CAD build for the part. Positions are in the model's coordinates, mm. Give positions to 0.01 mm unless a question says otherwise; leave off trailing zeros. Write each loop counter-clockwise with the first axis right and the second up, starting at its lowest first coordinate (ties: lowest second). Pieces come first, ordered by that corner, then holes. Notation, with made-up numbers: M 59.25,-4 L 77.25,-4 A27 cw 77.25,22 Z; hole C 2,6 d8. An arc over 180 degrees is marked long. One line per question, with ' | ' between items. Start each with the question number.
1. Wall check: L1, parallel to Y at x = -65, z = 2.1; L2, parallel to Y at x = -68.5, z = 1; L3, parallel to X at y = 59.5, z = 1. Give the ranges that are in metal, low to high.
2. Cut at C-C, the plane x = -58.5. Write the cut outline in (y, z).
3. Cut at B-B, the plane z = 5. Count the separate pieces of the cut face and the enclosed holes in it, then the cut area to 3 significant figures.
4. Cut at D-D, the plane y = 65. Write the cut outline in (x, z).
5. Flat gauge pins, fed straight in: pin 1 (1.5 mm diameter, centred on y = 38, z = 5, fed in from +X); pin 2 (5 mm diameter, centred on x = 65, y = -65, fed in from +Z); pin 3 (3 mm diameter, centred on x = -57.5, z = 5, fed in from -Y); pin 4 (1.5 mm diameter, centred on y = 2, z = 4, fed in from -X). Where does each tip first touch, or does it go through?
6. Cut at A-A, the plane y = 0. Write the cut outline in (x, z).
```python
from build123d import *

# Parameters (mm, degrees)
F0_R     = 4.25
F0_R_2   = 2.6
F1_DEPTH = 6
F2_R     = 20


with BuildPart() as f1:
    # F0 (on Top) → F1 (new body)
    with BuildSketch(Plane.XY):
        with BuildLine():
            Line((56.161165, 73.838835), (25.393825, 43.071495))
            ThreePointArc((25.393825, 43.071495), (0, 50), (-25.393825, 43.071495))
            Line((-25.393825, 43.071495), (-56.161165, 73.838835))
            ThreePointArc((-56.161165, 73.838835), (-73.838835, 73.838835), (-73.838835, 56.161165))
            Line((-73.838835, 56.161165), (-43.071495, 25.393825))
            ThreePointArc((-43.071495, 25.393825), (-50, 0), (-43.071495, -25.393825))
            Line((-43.071495, -25.393825), (-73.838835, -56.161165))
            ThreePointArc((-73.838835, -56.161165), (-73.838835, -73.838835), (-56.161165, -73.838835))
            Line((-56.161165, -73.838835), (-25.393825, -43.071495))
            ThreePointArc((-25.393825, -43.071495), (0, -50), (25.393825, -43.071495))
            Line((25.393825, -43.071495), (56.161165, -73.838835))
            ThreePointArc((56.161165, -73.838835), (73.838835, -73.838835), (73.838835, -56.161165))
            Line((73.838835, -56.161165), (43.071495, -25.393825))
            ThreePointArc((43.071495, -25.393825), (50, 0), (43.071495, 25.393825))
            Line((43.071495, 25.393825), (73.838835, 56.161165))
            ThreePointArc((73.838835, 56.161165), (73.838835, 73.838835), (56.161165, 73.838835))
        make_face()
        with Locations((-65, -65)):
            Circle(F0_R, mode=Mode.SUBTRACT)
        with Locations((65, -65)):
            Circle(F0_R, mode=Mode.SUBTRACT)
        with Locations((-32.5, 0)):
            Circle(F0_R_2, mode=Mode.SUBTRACT)
        with Locations((-65, 65)):
            Circle(F0_R, mode=Mode.SUBTRACT)
        with Locations((32.5, 0)):
            Circle(F0_R_2, mode=Mode.SUBTRACT)
        with Locations((65, 65)):
            Circle(F0_R, mode=Mode.SUBTRACT)
    extrude(amount=F1_DEPTH)

    # F2
    f2_edges = [f1.edges().sort_by_distance(p)[0] for p in [
        (-25.393825, -43.071495, 3),
        (25.393825, -43.071495, 3),
        (43.071495, -25.393825, 3),
        (43.071495, 25.393825, 3),
        (25.393825, 43.071495, 3),
        (-25.393825, 43.071495, 3),
        (-43.071495, 25.393825, 3),
        (-43.071495, -25.393825, 3),
    ]]
    fillet(f2_edges, radius=F2_R)


solid = f1.part
```
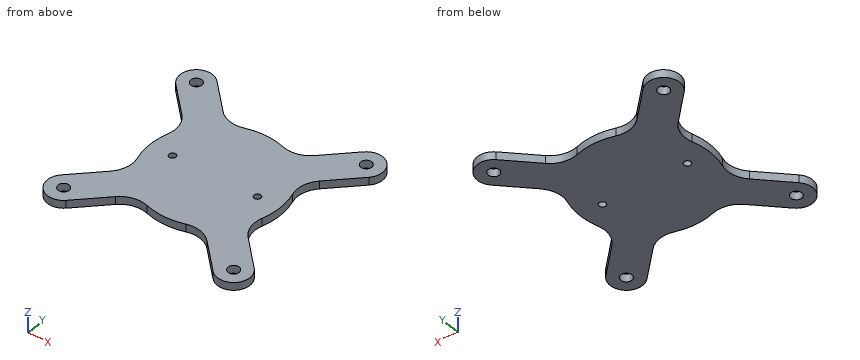
Here are the results:
1) L1: -77.5 to -69.25, -60.75 to -47.32, 47.32 to 60.75, 69.25 to 77.5 | L2: -77 to -67.41, -62.59 to -50.82, 50.82 to 62.59, 67.41 to 77 | L3: -76.22 to -41.82, 41.82 to 76.22
2) outline: M -75.68,0 L -40.82,0 L -40.82,6 L -75.68,6 Z; M 40.82,0 L 75.68,0 L 75.68,6 L 40.82,6 Z
3) separate pieces: 1 | enclosed holes: 6 | area: 13,000 mm^2
4) outline: M -77.5,0 L -69.25,0 L -69.25,6 L -77.5,6 Z; M -60.75,0 L -47.32,0 L -47.32,6 L -60.75,6 Z; M 47.32,0 L 60.75,0 L 60.75,6 L 47.32,6 Z; M 69.25,0 L 77.5,0 L 77.5,6 L 69.25,6 Z
5) pin 1: x = 56.43 | pin 2: through | pin 3: y = -75.97 | pin 4: x = -49.98
6) outline: M -50,0 L -35.1,0 L -35.1,6 L -50,6 Z; M -29.9,0 L 29.9,0 L 29.9,6 L -29.9,6 Z; M 35.1,0 L 50,0 L 50,6 L 35.1,6 Z
